from build123d import *

# Parameters (mm, degrees)
F0_R     = 2.5
F0_R_2   = 1.5
F1_DEPTH = 4


with BuildPart() as f1:
    # F0 (on Top) → F1 (new body)
    with BuildSketch(Plane.XY):
        with BuildLine():
            ThreePointArc((100, 36.7082039325), (99.5643546459, 38.7494453848), (98.3333333333, 40.434983895))
            ThreePointArc((98.3333333333, 40.434983895), (88.2480547914, 43.9797917868), (78.6012006129, 39.3736317032))
            add(Edge.make_bspline(
                [(78.2678444341, 38.9900409849), (78.3796218574, 39.1174296296), (78.4907435172, 39.2452925352), (78.6012006129, 39.3736317032)],
                knots=[0.9951145834, 0.9951145834, 0.9951145834, 0.9951145834, 1, 1, 1, 1], degree=3))
            ThreePointArc((78.2678444341, 38.9900409849), (76.230411331, 24.2608706912), (88.5978294237, 16.0057776626))
            ThreePointArc((88.5978294237, 16.0057776626), (93.807126129, 16.8511773006), (98.3333333333, 19.565016105))
            ThreePointArc((98.3333333333, 19.565016105), (99.5643546459, 21.2505546152), (100, 23.2917960675))
            Line((100, 23.2917960675), (100, 36.7082039325))
        make_face()
        with BuildLine():
            Line((86.490440342, 24.8812003045), (83.846652322, 21.8794699859))
            ThreePointArc((83.846652322, 21.8794699859), (82.8159172375, 21.3738963808), (81.729582945, 21.745241624))
            ThreePointArc((81.729582945, 21.745241624), (81.2240093398, 22.7759767085), (81.595354583, 23.8623110009))
            Line((81.595354583, 23.8623110009), (84.239142603, 26.8640413195))
            ThreePointArc((84.239142603, 26.8640413195), (85.2698776875, 27.3696149247), (86.35621198, 26.9982696815))
            ThreePointArc((86.35621198, 26.9982696815), (86.8617855852, 25.967534597), (86.490440342, 24.8812003045))
        make_face(mode=Mode.SUBTRACT)
        with BuildLine():
            Line((94.1187996955, 27.490440342), (97.1205300141, 24.846652322))
            ThreePointArc((97.1205300141, 24.846652322), (97.6261036192, 23.8159172375), (97.254758376, 22.729582945))
            ThreePointArc((97.254758376, 22.729582945), (96.2240232915, 22.2240093398), (95.1376889991, 22.595354583))
            Line((95.1376889991, 22.595354583), (92.1359586805, 25.239142603))
            ThreePointArc((92.1359586805, 25.239142603), (91.6303850753, 26.2698776875), (92.0017303185, 27.35621198))
            ThreePointArc((92.0017303185, 27.35621198), (93.032465403, 27.8617855852), (94.1187996955, 27.490440342))
        make_face(mode=Mode.SUBTRACT)
        with Locations((89, 30)):
            Circle(F0_R, mode=Mode.SUBTRACT)
        with BuildLine():
            Line((83.8812003045, 32.509559658), (80.8794699859, 35.153347678))
            ThreePointArc((80.8794699859, 35.153347678), (80.3738963808, 36.1840827625), (80.745241624, 37.270417055))
            ThreePointArc((80.745241624, 37.270417055), (81.7759767085, 37.7759906602), (82.8623110009, 37.404645417))
            Line((82.8623110009, 37.404645417), (85.8640413195, 34.760857397))
            ThreePointArc((85.8640413195, 34.760857397), (86.3696149247, 33.7301223125), (85.9982696815, 32.64378802))
            ThreePointArc((85.9982696815, 32.64378802), (84.967534597, 32.1382144148), (83.8812003045, 32.509559658))
        make_face(mode=Mode.SUBTRACT)
        with BuildLine():
            Line((91.509559658, 35.1187996955), (94.153347678, 38.1205300141))
            ThreePointArc((94.153347678, 38.1205300141), (95.1840827625, 38.6261036192), (96.270417055, 38.254758376))
            ThreePointArc((96.270417055, 38.254758376), (96.7759906602, 37.2240232915), (96.404645417, 36.1376889991))
            Line((96.404645417, 36.1376889991), (93.760857397, 33.1359586805))
            ThreePointArc((93.760857397, 33.1359586805), (92.7301223125, 32.6303850753), (91.64378802, 33.0017303185))
            ThreePointArc((91.64378802, 33.0017303185), (91.1382144148, 34.032465403), (91.509559658, 35.1187996955))
        make_face(mode=Mode.SUBTRACT)
        with BuildLine():
            add(Edge.make_bspline(
                [(78.2678444341, 38.9900409849), (78.3796218574, 39.1174296296), (78.4907435172, 39.2452925352), (78.6012006129, 39.3736317032)],
                knots=[0.9951145834, 0.9951145834, 0.9951145834, 0.9951145834, 1, 1, 1, 1], degree=3))
            ThreePointArc((78.6012006129, 39.3736317032), (78.4327818341, 39.1833490751), (78.2678444341, 38.9900409849))
        make_face()
        with BuildLine():
            ThreePointArc((88.5978294237, 16.0057776626), (76.230411331, 24.2608706912), (78.2678444341, 38.9900409849))
            add(Edge.make_bspline(
                [(0, 4.748087842), (3.7510812941, 4.556623698), (23.9631634822, 9.0849893596), (63.9002947469, 22.6158696289), (78.2678444341, 38.9900409849)],
                knots=[0, 0, 0, 0, 0.3671571365, 0.9951145834, 0.9951145834, 0.9951145834, 0.9951145834], degree=3))
            add(Edge.make_bspline(
                [(0, 4.748087842), (-3.7510812941, 4.556623698), (-23.9631634822, 9.0849893596), (-63.9002947469, 22.6158696289), (-78.2678444341, 38.9900409849)],
                knots=[0, 0, 0, 0, 0.3671571365, 0.9951145834, 0.9951145834, 0.9951145834, 0.9951145834], degree=3))
            ThreePointArc((-78.2678444341, 38.9900409849), (-76.230411331, 24.2608706912), (-88.5978294237, 16.0057776626))
            add(Edge.make_bspline(
                [(0, -20), (-3.7175141039, -19.8114133897), (-24.2979575574, -32.2702358468), (-52.3226244724, 16.7220671125), (-88.5978294237, 16.0057776626)],
                knots=[0, 0, 0, 0, 0.3194759338, 1, 1, 1, 1], degree=3))
            add(Edge.make_bspline(
                [(0, -20), (3.7175141039, -19.8114133897), (24.2979575574, -32.2702358468), (52.3226244724, 16.7220671125), (88.5978294237, 16.0057776626)],
                knots=[0, 0, 0, 0, 0.3194759338, 1, 1, 1, 1], degree=3))
        make_face()
        with Locations((-14.5, -17)):
            Circle(F0_R_2, mode=Mode.SUBTRACT)
        with Locations((-22, 0)):
            Circle(F0_R_2, mode=Mode.SUBTRACT)
        with Locations((14.5, -17)):
            Circle(F0_R_2, mode=Mode.SUBTRACT)
        with Locations((22, 0)):
            Circle(F0_R_2, mode=Mode.SUBTRACT)
        with BuildLine():
            add(Edge.make_bspline(
                [(-78.2678444341, 38.9900409849), (-78.3796218574, 39.1174296296), (-78.4907435172, 39.2452925352), (-78.6012006129, 39.3736317032)],
                knots=[0.9951145834, 0.9951145834, 0.9951145834, 0.9951145834, 1, 1, 1, 1], degree=3))
            ThreePointArc((-78.2678444341, 38.9900409849), (-78.4327818341, 39.1833490751), (-78.6012006129, 39.3736317032))
        make_face()
        with BuildLine():
            ThreePointArc((-88.5978294237, 16.0057776626), (-76.230411331, 24.2608706912), (-78.2678444341, 38.9900409849))
            add(Edge.make_bspline(
                [(-78.2678444341, 38.9900409849), (-78.3796218574, 39.1174296296), (-78.4907435172, 39.2452925352), (-78.6012006129, 39.3736317032)],
                knots=[0.9951145834, 0.9951145834, 0.9951145834, 0.9951145834, 1, 1, 1, 1], degree=3))
            ThreePointArc((-78.6012006129, 39.3736317032), (-88.2480547914, 43.9797917868), (-98.3333333333, 40.434983895))
            ThreePointArc((-98.3333333333, 40.434983895), (-99.5643546459, 38.7494453848), (-100, 36.7082039325))
            Line((-100, 36.7082039325), (-100, 23.2917960675))
            ThreePointArc((-100, 23.2917960675), (-99.5643546459, 21.2505546152), (-98.3333333333, 19.565016105))
            ThreePointArc((-98.3333333333, 19.565016105), (-93.807126129, 16.8511773006), (-88.5978294237, 16.0057776626))
        make_face()
        with BuildLine():
            ThreePointArc((-81.729582945, 21.745241624), (-82.8159172375, 21.3738963808), (-83.846652322, 21.8794699859))
            Line((-83.846652322, 21.8794699859), (-86.490440342, 24.8812003045))
            ThreePointArc((-86.490440342, 24.8812003045), (-86.8617855852, 25.967534597), (-86.35621198, 26.9982696815))
            ThreePointArc((-86.35621198, 26.9982696815), (-85.2698776875, 27.3696149247), (-84.239142603, 26.8640413195))
            Line((-84.239142603, 26.8640413195), (-81.595354583, 23.8623110009))
            ThreePointArc((-81.595354583, 23.8623110009), (-81.2240093398, 22.7759767085), (-81.729582945, 21.745241624))
        make_face(mode=Mode.SUBTRACT)
        with BuildLine():
            Line((-92.1359586805, 25.239142603), (-95.1376889991, 22.595354583))
            ThreePointArc((-95.1376889991, 22.595354583), (-96.2240232915, 22.2240093398), (-97.254758376, 22.729582945))
            ThreePointArc((-97.254758376, 22.729582945), (-97.6261036192, 23.8159172375), (-97.1205300141, 24.846652322))
            Line((-97.1205300141, 24.846652322), (-94.1187996955, 27.490440342))
            ThreePointArc((-94.1187996955, 27.490440342), (-93.032465403, 27.8617855852), (-92.0017303185, 27.35621198))
            ThreePointArc((-92.0017303185, 27.35621198), (-91.6303850753, 26.2698776875), (-92.1359586805, 25.239142603))
        make_face(mode=Mode.SUBTRACT)
        with Locations((-89, 30)):
            Circle(F0_R, mode=Mode.SUBTRACT)
        with BuildLine():
            Line((-93.760857397, 33.1359586805), (-96.404645417, 36.1376889991))
            ThreePointArc((-96.404645417, 36.1376889991), (-96.7759906602, 37.2240232915), (-96.270417055, 38.254758376))
            ThreePointArc((-96.270417055, 38.254758376), (-95.1840827625, 38.6261036192), (-94.153347678, 38.1205300141))
            Line((-94.153347678, 38.1205300141), (-91.509559658, 35.1187996955))
            ThreePointArc((-91.509559658, 35.1187996955), (-91.1382144148, 34.032465403), (-91.64378802, 33.0017303185))
            ThreePointArc((-91.64378802, 33.0017303185), (-92.7301223125, 32.6303850753), (-93.760857397, 33.1359586805))
        make_face(mode=Mode.SUBTRACT)
        with BuildLine():
            ThreePointArc((-80.745241624, 37.270417055), (-80.3738963808, 36.1840827625), (-80.8794699859, 35.153347678))
            Line((-80.8794699859, 35.153347678), (-83.8812003045, 32.509559658))
            ThreePointArc((-83.8812003045, 32.509559658), (-84.967534597, 32.1382144148), (-85.9982696815, 32.64378802))
            ThreePointArc((-85.9982696815, 32.64378802), (-86.3696149247, 33.7301223125), (-85.8640413195, 34.760857397))
            Line((-85.8640413195, 34.760857397), (-82.8623110009, 37.404645417))
            ThreePointArc((-82.8623110009, 37.404645417), (-81.7759767085, 37.7759906602), (-80.745241624, 37.270417055))
        make_face(mode=Mode.SUBTRACT)
    extrude(amount=F1_DEPTH)


solid = f1.part
The model under review builds one solid part; all positions refer to its coordinate system, in mm. Give positions to 0.01 mm unless a question says otherwise; leave off trailing zeros.
1. Draft analysis for pull direction X (two halves, no side actions). For faces 1 (the cylindrical face through (99.576, 38.723, 1.972)), 2 (the cylindrical face through (-99.576, 21.277, 1.972)), 3 (the cylindrical face through (87.16, 31.69, 1.97)), state which applies: +X half, -X half, draft (parallel to the pull), parting line (faces both ways), or undercut.
2. For P1, Ø8, axis at x = 89, y = 30, coming from the -Z side; P2, Ø2, axis at x = -4, z = 2, coming from the -Y side; P3, Ø1.5, axis at y = 3.5, z = 3, coming from the +X side, all flat-tipped, find the tip position at first contact; note any pin that passes through.
3. Wall thickness on L1, parallel to Y at x = -89, z = 0.95; L2, parallel to X at y = 22, z = 3.75; L3, parallel to X at y = 18, z = 3: over which ranges is each line inside the solid? List them lowest first.
4. Add section A-A, the plane z = 1.8. Count the separate pieces of the cut face and the enclosed holes in it, plus the area to 3 significant figures.
Worked answers:
1. face 1: +X half
1. face 2: -X half
1. face 3: undercut
2. P1: stops at z = 0
2. P2: stops at y = -20.92
2. P3: stops at x = 52.04
3. L1: y = 16 to 27.5, 32.5 to 44
3. L2: x = -99.83 to -83.95, -81.5 to -55.45, 55.45 to 81.5, 83.95 to 99.83
3. L3: x = -96.21 to -46.97, 46.97 to 96.21
4. separate pieces: 1
4. enclosed holes: 14
4. area: 4,360 mm2
